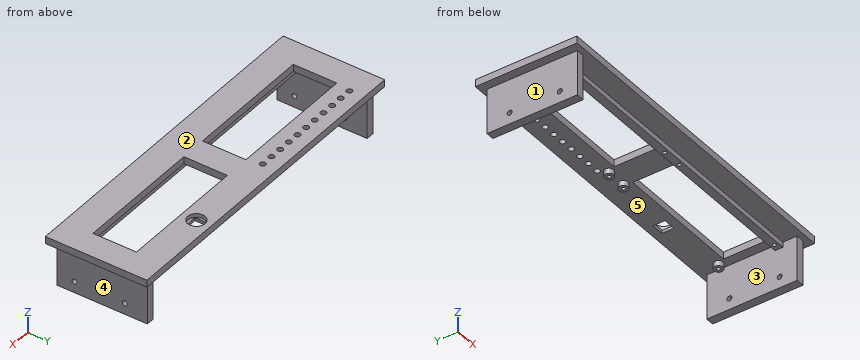
from build123d import *

# Parameters (mm, degrees)
SKETCH_W      = 187.325
SKETCH_H      = 57.15
SKETCH_R      = 1.5875
SKETCH_W_2    = 71.6026
SKETCH_H_2    = 24.4602
PAD_DEPTH     = 4.0132
SKETCH001_R   = 2.54
SKETCH001_R_2 = 1.016
SKETCH001_W   = 168.656
SKETCH001_H   = 4.445
PAD001_DEPTH  = 2.921
SKETCH002_W   = 4.572
SKETCH002_H   = 50.8
PAD002_DEPTH  = 25.4
SKETCH003_R   = 1.389063
HOLE_DEPTH    = 177.8
HOLE_TIPS_R   = 1.389063
SKETCH004_R   = 4.8895
HOLE001_DEPTH = 2.286
SKETCH005_W   = 7.112
SKETCH005_H   = 6.711802
POCKET_DEPTH  = 27.1282


with BuildPart() as part:
    # Sketch → Pad (new body)
    with BuildSketch(Plane.XY):
        Rectangle(SKETCH_W, SKETCH_H)
        with Locations((-77.338766, 20.40255)):
            Circle(SKETCH_R, mode=Mode.SUBTRACT)
        with Locations((-70.516326, 20.40255)):
            Circle(SKETCH_R, mode=Mode.SUBTRACT)
        with Locations((-63.693886, 20.40255)):
            Circle(SKETCH_R, mode=Mode.SUBTRACT)
        with Locations((-56.871446, 20.40255)):
            Circle(SKETCH_R, mode=Mode.SUBTRACT)
        with Locations((-50.049006, 20.40255)):
            Circle(SKETCH_R, mode=Mode.SUBTRACT)
        with Locations((-43.226566, 20.40255)):
            Circle(SKETCH_R, mode=Mode.SUBTRACT)
        with Locations((-36.404126, 20.40255)):
            Circle(SKETCH_R, mode=Mode.SUBTRACT)
        with Locations((-29.581686, 20.40255)):
            Circle(SKETCH_R, mode=Mode.SUBTRACT)
        with Locations((-22.759246, 20.40255)):
            Circle(SKETCH_R, mode=Mode.SUBTRACT)
        with Locations((-15.936806, 20.40255)):
            Circle(SKETCH_R, mode=Mode.SUBTRACT)
        with Locations((-9.114366, 20.40255)):
            Circle(SKETCH_R, mode=Mode.SUBTRACT)
        with Locations((43.213867, 0)):
            Rectangle(SKETCH_W_2, SKETCH_H_2, mode=Mode.SUBTRACT)
        with Locations((-43.036066, 0)):
            Rectangle(SKETCH_W_2, SKETCH_H_2, mode=Mode.SUBTRACT)
    extrude(amount=PAD_DEPTH)

    # Sketch001 (on Face24 of Pad) → Pad001 (join)
    with BuildSketch(Plane(origin=(0, 0, 0), x_dir=(1, 0, 0), z_dir=(0, 0, -1))):
        with Locations((80.666167, -16.1925)):
            Circle(SKETCH001_R)
        with Locations((80.666167, -16.1925)):
            Circle(SKETCH001_R_2, mode=Mode.SUBTRACT)
        with Locations((5.761567, -16.1925)):
            Circle(SKETCH001_R)
        with Locations((5.761567, -16.1925)):
            Circle(SKETCH001_R_2, mode=Mode.SUBTRACT)
        with Locations((-5.583766, -16.1925)):
            Circle(SKETCH001_R)
        with Locations((-5.583766, -16.1925)):
            Circle(SKETCH001_R_2, mode=Mode.SUBTRACT)
        with Locations((-80.488366, -16.1925)):
            Circle(SKETCH001_R)
        with Locations((-80.488366, -16.1925)):
            Circle(SKETCH001_R_2, mode=Mode.SUBTRACT)
        with Locations((0, 15.1257)):
            Rectangle(SKETCH001_W, SKETCH001_H)
        with Locations((-80.488366, 15.1257)):
            Circle(SKETCH001_R_2, mode=Mode.SUBTRACT)
        with Locations((-5.583766, 15.1257)):
            Circle(SKETCH001_R_2, mode=Mode.SUBTRACT)
        with Locations((5.761567, 15.1257)):
            Circle(SKETCH001_R_2, mode=Mode.SUBTRACT)
        with Locations((80.666167, 15.1257)):
            Circle(SKETCH001_R_2, mode=Mode.SUBTRACT)
    extrude(amount=PAD001_DEPTH)

    # Sketch002 (on Face4 of Pad001) → Pad002 (join)
    with BuildSketch(Plane(origin=(0, 0, 0), x_dir=(1, 0, 0), z_dir=(0, 0, -1))):
        with Locations((86.614, 0)):
            Rectangle(SKETCH002_W, SKETCH002_H)
        with Locations((-86.614, 0)):
            Rectangle(SKETCH002_W, SKETCH002_H)
    extrude(amount=PAD002_DEPTH)

    # Sketch003 (on Face15 of Pad002) → Hole (cut)
    with BuildSketch(Plane(origin=(-88.9, 0, 0), x_dir=(0, -1, 0), z_dir=(-1, 0, 0))):
        with Locations((-12.7, -19.05)):
            Circle(SKETCH003_R)
        with Locations((15.56766, -19.05)):
            Circle(SKETCH003_R)
    extrude(amount=-HOLE_DEPTH, mode=Mode.SUBTRACT)

    # Hole tips → Hole tip 1 section 0
    with BuildSketch(Plane(origin=(88.9, 0, 0), x_dir=(0, -1, 0), z_dir=(-1, 0, 0)), mode=Mode.PRIVATE) as hole_tip_1_s0:
        with Locations((-12.7, -19.05)):
            Circle(HOLE_TIPS_R)
    loft([hole_tip_1_s0.sketch, Vertex(89.734633, 12.7, -19.05)], mode=Mode.SUBTRACT)

    # Hole tips → Hole tip 2 section 0
    with BuildSketch(Plane(origin=(88.9, 0, 0), x_dir=(0, -1, 0), z_dir=(-1, 0, 0)), mode=Mode.PRIVATE) as hole_tip_2_s0:
        with Locations((15.56766, -19.05)):
            Circle(HOLE_TIPS_R)
    loft([hole_tip_2_s0.sketch, Vertex(89.734633, -15.56766, -19.05)], mode=Mode.SUBTRACT)

    # Sketch004 (on Face5 of Hole) → Hole001 (cut)
    with BuildSketch(Plane.XY.offset(4.0132)):
        with Locations((43.213867, 20.40255)):
            Circle(SKETCH004_R)
    extrude(amount=-HOLE001_DEPTH, mode=Mode.SUBTRACT)

    # Sketch005 (on Face52 of Hole001) → Pocket (cut, through all)
    with BuildSketch(Plane.XY.offset(1.7272)):
        with Locations((43.213867, 20.40255)):
            Rectangle(SKETCH005_W, SKETCH005_H)
    extrude(amount=-POCKET_DEPTH, mode=Mode.SUBTRACT)


solid = part.part
For this review, take the finished solid that the model builds, in its own axes (mm). Face numbers are marked on the shaded views. A direction names the side the tool comes from. Round coordinates to 2 decimals unless told otherwise and drop trailing zeros. Write each loop counter-clockwise with the first axis right and the second up, starting at its lowest first coordinate (ties: lowest second). Pieces come first, ordered by that corner, then holes. Notation, with made-up numbers: M 87,6 L 126,6 A15 cw 126,30 Z; hole C 89.5,-34 d10. An arc over 180 degrees is marked long. Write item = value, one per line. Start each with the question number.
(1) We need section A-A (x = 68). Give the boundary of the cut face in (y, z) (3 decimals).
(2) Clearance check with flat-ended pins moving along their axes: pin 1 Ø6 at (x, y) = (30, 12) entering from -Z; pin 2 Ø8 at (y, z) = (10.5, -22) entering from -X; pin 3 Ø0.8 at (x, y) = (42.5, 24.5) entering from +Z. State where each tip first meets the part, or that it passes through.
(3) We need section D-D (x = 42.5). Give the boundary of the cut face in (y, z) (3 decimals).
(4) For the marked faces 4 and 5, list the 3-axis set-ups (+Z, -Z, +X, -X, +Y, -Y) from which the entire face can be reached by the end or side of a thin tool; tool diameter is ignored.
(5) The part is to be moulded in two halves that separate along X. For the marked faces 1, 2 and 3, say which applies: +X half, -X half, draft (parallel to the pull), parting line (faces both ways), or undercut.
(6) We need section B-B (y = 3). Give the boundary of the cut face in (x, z).
(7) We need section C-C (z = -5.5). Give the boundary of the cut face in (x, y), then the cut area to 3 significant figures.
(8) For line 1 along X through (y, z) = (-7, 0.5); line 2 along X through (y, z) = (-4, -22.25); line 3 along Z through (x, y) = (-39, -16.5), list the stretches that pass through material, from the lowest coordinate up.
Results found:
q1.outline = M -28.575,0 L -17.348,0 L -17.348,-2.921 L -12.903,-2.921 L -12.903,0 L -12.23,0 L -12.23,4.013 L -28.575,4.013 Z; M 12.23,0 L 28.575,0 L 28.575,4.013 L 12.23,4.013 Z
q2.pin_1 = 0
q2.pin_2 = -88.9
q2.pin_3 = 1.73
q3.outline = M -28.575,0 L -17.348,0 L -17.348,-2.921 L -12.903,-2.921 L -12.903,0 L -12.23,0 L -12.23,4.013 L -28.575,4.013 Z; M 12.23,0 L 17.047,0 L 17.047,1.727 L 15.565,1.727 L 15.565,4.013 L 12.23,4.013 Z; M 23.758,0 L 28.575,0 L 28.575,4.013 L 25.24,4.013 L 25.24,1.727 L 23.758,1.727 Z
q4.face_4 = -Z, +X, +Y, -Y
q4.face_5 = -Z
q5.face_1 = -X half
q5.face_2 = draft
q5.face_3 = undercut
q6.outline = M -93.66,0 L -88.9,0 L -88.9,-25.4 L -84.33,-25.4 L -84.33,0 L -78.84,0 L -78.84,4.01 L -93.66,4.01 Z; M -7.23,0 L 7.41,0 L 7.41,4.01 L -7.23,4.01 Z; M 79.02,0 L 84.33,0 L 84.33,-25.4 L 88.9,-25.4 L 88.9,0 L 93.66,0 L 93.66,4.01 L 79.02,4.01 Z
q7.outline = M -88.9,-25.4 L -84.33,-25.4 L -84.33,25.4 L -88.9,25.4 Z; M 84.33,-25.4 L 88.9,-25.4 L 88.9,25.4 L 84.33,25.4 Z
q7.area = 465 mm²
q8.line_1 = -93.66 to -78.84, -7.23 to 7.41, 79.02 to 93.66
q8.line_2 = -88.9 to -84.33, 84.33 to 88.9
q8.line_3 = -2.92 to 4.01
